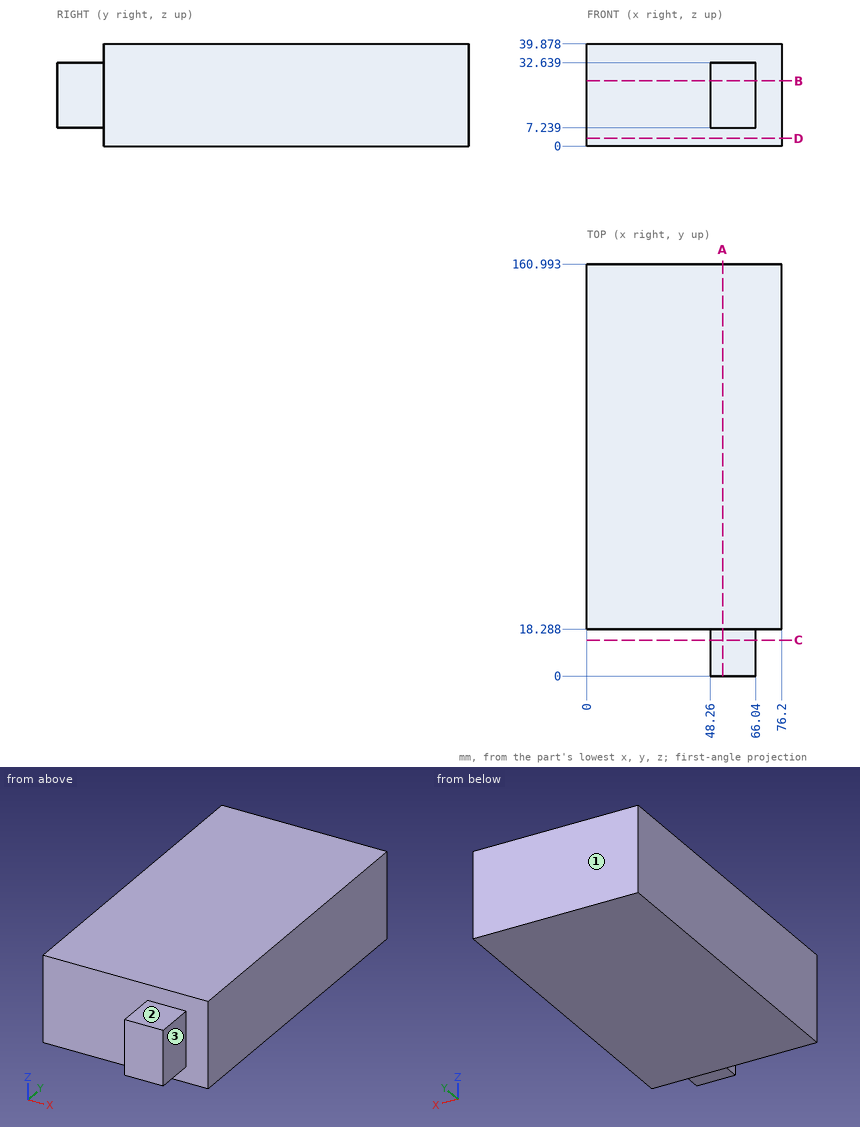
Here's the drawing with two shaded views (mm, measured from the low corner). I have some questions. A direction names the side the tool comes from. Give positions to 0.01 mm unless a question says otherwise; leave off trailing zeros. Write each loop counter-clockwise with the first axis right and the second up, starting at its lowest first coordinate (ties: lowest second). Pieces come first, ordered by that corner, then holes. Notation, with made-up numbers: (-6, 18.5) -> (18, 18.5) arc R13 cw to (18, 27.5) -> close; hole circle Ø4 at (24, -32.5). An arc over 180 degrees is marked (long way). Answer as a JSON object with one key per item and string values. Group by question number.
Item 1: For the marked faces 1, 2 and 3, which set-ups out of +Z, -Z, +X, -X, +Y, -Y let a thin tool reach every point of the face, with its end or its side?
Item 2: Suppose I cut it at D-D (z = 3). Please give me the cut outline in (x, y).
Item 3: Suppose I cut it at B-B (z = 25.5). Please give me the cut outline in (x, y).
Item 4: I'm going to push flat-ended pins straight in: P1, Ø19.5, axis at x = 60, y = 8, coming from the +Z side; P2, Ø9, axis at y = 8, z = 21.5, coming from the +X side; P3, Ø2, axis at x = 18, z = 26, coming from the -Y side. Where does each tip first touch, or does it pass through?
Item 5: Please list where these lines run through material, in increasing order: line 1 (Y direction, x = 49, z = 35.5); line 2 (X direction, y = 17.5, z = 13). Write a range as [from, to].
Item 6: Suppose I cut it at A-A (x = 53). Please give me the cut outline in (y, z), plus the area to 3 significant figures.
Item 7: Suppose I cut it at C-C (y = 14). Please give me the cut outline in (x, z).
Findings:
{
 "1": {"face 1": "+Z, -Z, +X, -X, +Y", "face 2": "+Z, +X, -X, -Y", "face 3": "+Z, -Z, +X, -Y"},
 "2": {"outline": "(0, 18.29) -> (76.2, 18.29) -> (76.2, 160.99) -> (0, 160.99) -> close"},
 "3": {"outline": "(0, 18.29) -> (48.26, 18.29) -> (48.26, 0) -> (66.04, 0) -> (66.04, 18.29) -> (76.2, 18.29) -> (76.2, 160.99) -> (0, 160.99) -> close"},
 "4": {"P1": "stops at z = 32.64", "P2": "stops at x = 66.04", "P3": "stops at y = 18.29"},
 "5": {"line 1": "y = [18.29, 160.99]", "line 2": "x = [48.26, 66.04]"},
 "6": {"outline": "(0, 7.24) -> (18.29, 7.24) -> (18.29, 0) -> (160.99, 0) -> (160.99, 39.88) -> (18.29, 39.88) -> (18.29, 32.64) -> (0, 32.64) -> close", "area": "6,160 mm²"},
 "7": {"outline": "(48.26, 7.24) -> (66.04, 7.24) -> (66.04, 32.64) -> (48.26, 32.64) -> close"}
}
